Source: CAD feature listing. Evaluate the final solid. Frame: model axes, mm. Give positions to 0.01 mm unless a question says otherwise; leave off trailing zeros. Order: outer loops, then holes, each group sorted by start corner. A loop starts at its lowest first (then second) coordinate and runs counter-clockwise, first axis right, second up. Notation, with made-up numbers: (-16.75, -0.75) -> (-3.75, -0.75) arc R10 cw to (-3.75, 5.25) -> close; hole circle Ø7 at (41.25, 9.5). An arc over 180 degrees is marked (long way). Answer in a Markdown table with one row per item.
Autodesk Inventor part; units mm, degrees
ref_plane "YZ Plane" through (0, 0, 0) normal (1, 0, 0) x (0, 1, 0)
ref_plane "XZ Plane" through (0, 0, 0) normal (0, 1, 0) x (-1, 0, 0)
ref_plane "XY Plane" through (0, 0, 0) normal (0, 0, 1) x (1, 0, 0)
sketch "Sketch1" plane through (0, 0, 0) normal (0, 0, 1) x (1, 0, 0)
  line L0 (-50.8, -28.575) -> (50.8, -28.575)
  line L1 (50.8, -28.575) -> (50.8, 28.575)
  line L2 (50.8, 28.575) -> (-50.8, 28.575)
  line L3 (-50.8, 28.575) -> (-50.8, -28.575)
  line L4 (-50.8, -28.575) -> (50.8, 28.575) construction
  line L5 (50.8, -28.575) -> (-50.8, 28.575) construction
  circle A0 centre (-46.99, 24.765) radius 1.4
  line L6 (-50.8, 0) -> (50.8, 0) construction
  line L7 (0, 28.575) -> (0, -28.575) construction
  circle A1 centre (-46.99, -24.765) radius 1.4
  circle A2 centre (46.99, 24.765) radius 1.4
  circle A3 centre (46.99, -24.765) radius 1.4
  circle A4 centre (-26.67, 24.765) radius 1.4
  circle A5 centre (26.67, 24.765) radius 1.4
  circle A6 centre (-26.67, -24.765) radius 1.4
  circle A7 centre (26.67, -24.765) radius 1.4
  point P0 (0, 0)
  dimension "d2" = 101.6
  dimension "d4" = 57.15
  dimension "d5" = 49.53
  dimension "d6" = 2.8
  dimension "d8" = 2.8
  dimension "d10" = 49.53
  dimension "d21" = 3.81
  dimension "d22" = 3.81
  dimension "d23" = 3.81
  dimension "d24" = 3.81
  dimension "d25" = 3.81
  dimension "d26" = 3.81
  dimension "d27" = 3.81
  dimension "d28" = 3.81
  dimension "d29" = 20.32
  dimension "d30" = 53.34
  dimension "d31" = 49.53
  dimension "d32" = 93.98
extrude "Extrusion1" add sketch "Sketch1" along normal blind 1 contours L3 L2 L1 L0 | A4 | A5 | A6 | A7
sketch "Sketch3" plane through (0, 0, 1) normal (0, 0, 1) x (1, 0, 0)
  circle A0 centre (26.67, -24.765) radius 1.4
  circle A1 centre (-26.67, -24.765) radius 1.4
  line L0 (50.8, 28.575) -> (-50.8, 28.575)
  line L1 (-21.67, -25.765) -> (21.67, -25.765)
  line L2 (21.67, -25.765) -> (21.67, 30.575)
  line L3 (21.67, 30.575) -> (-21.67, 30.575)
  line L4 (-21.67, 30.575) -> (-21.67, -25.765)
  line L5 (50.8, -28.575) -> (50.8, 28.575)
  line L6 (-50.8, 28.575) -> (-50.8, -28.575)
  point P0 (0, 0)
  dimension "d15" = 2
  dimension "d16" = 5
  dimension "d17" = 5
  dimension "d18" = 1
  dimension "d33" = 29.13
  dimension "d34" = 29.13
extrude "Extrusion3" [suppressed]
properties part number "PCB01" material "PCB(1)"
(1) Section query A-A (x = 46.99). Return the cut outline in (y, z) (3 decimals), plus the area to 4 significant figures.
A:
| item | result |
|---|---|
| outline | (-28.575, 0) -> (-26.165, 0) -> (-26.165, 1) -> (-28.575, 1) -> close; (-23.365, 0) -> (23.365, 0) -> (23.365, 1) -> (-23.365, 1) -> close; (26.165, 0) -> (28.575, 0) -> (28.575, 1) -> (26.165, 1) -> close |
| area | 51.55 mm^2 |
(2) Pull-direction query (X, two-part tool) for faces 1 (the cylindrical face through (-45.655, 24.344, 0.493)), 2 (the flat face through (-1, 0, 1)), 3 (the cylindrical face through (48.325, -25.186, 0.493)); classes: +X half, -X half, draft (parallel to the pull), parting line (faces both ways), or undercut.
A:
| item | result |
|---|---|
| face 1 | undercut |
| face 2 | draft |
| face 3 | undercut |
(3) Ray query, probe 1 along Y at (x, z) = (-46.99, 0.65) (3 decimals). Return the intervals inside material, ascending.
A:
| item | result |
|---|---|
| probe 1 | y = -28.575 to -26.165, -23.365 to 23.365, 26.165 to 28.575 |
